Input: part model. Units: mm. Frame: model coordinates. A direction names the side the tool comes from. Give positions to 0.01 mm unless a question says otherwise; leave off trailing zeros. Loops run counter-clockwise (first coordinate to the right, second up) from the corner with the lowest first, then second, coordinate; pieces in that order, holes last. Notation, with made-up numbers: (56, 21) -> (75, 21) arc R20 cw to (75, 36) -> close; hole circle Ø5 at (85, 49.25). An arc over 180 degrees is marked (long way). Answer as a JSON object with one key per item and string values.
```python
from build123d import *

# Parameters (mm, degrees)
SKETCH1_R           = 60
BOSS_EXTRUDE1_DEPTH = 3
SKETCH2_R           = 7.4
CUT_EXTRUDE3_DEPTH  = 85.905830189
CUT_EXTRUDE1_START  = -3
SKETCH3_W           = 3
SKETCH3_H           = 65
CUT_EXTRUDE1_DEPTH  = 3
SKETCH4_W           = 5
SKETCH4_H           = 5
SKETCH4_W_2         = 5.5
SKETCH4_H_2         = 8.5
CUT_EXTRUDE2_DEPTH  = 3
SKETCH6_R           = 2
CUT_EXTRUDE4_DEPTH  = 77.896033708


with BuildPart() as part:
    # Sketch1 → Boss-Extrude1 (new body)
    with BuildSketch(Plane(origin=(0, 0, 0), x_dir=(1, 0, 0), z_dir=(0, 1, 0))):
        with Locations(Location((0, 0, 0), (0, 0, 270))):
            Circle(SKETCH1_R)
    extrude(amount=BOSS_EXTRUDE1_DEPTH)

    # Sketch2 → Cut-Extrude3 (cut, through all)
    with BuildSketch(Plane(origin=(0, 3, 0), x_dir=(1, 0, 0), z_dir=(0, 1, 0))):
        with Locations(Location((0, 0, 0), (0, 0, 270))):
            Circle(SKETCH2_R)
    extrude(amount=-CUT_EXTRUDE3_DEPTH, mode=Mode.SUBTRACT)

    # Sketch3 → Cut-Extrude1 (cut)
    with BuildSketch(Plane(origin=(0, 3, 0), x_dir=(1, 0, 0), z_dir=(0, 1, 0)).offset(CUT_EXTRUDE1_START)):
        with Locations((-46.5, 0)):
            Rectangle(SKETCH3_W, SKETCH3_H)
        with BuildLine():
            Line((-48, 32.5), (-48, 36))
            ThreePointArc((-48, 36), (-60, 0), (-48, -36))
            Line((-48, -36), (-48, -32.5))
            Line((-48, -32.5), (-48, 32.5))
        make_face()
    cut_extrude1 = extrude(amount=CUT_EXTRUDE1_DEPTH, mode=Mode.SUBTRACT)

    # Sketch4 → Cut-Extrude2 (cut)
    with BuildSketch(Plane(origin=(0, 3, 0), x_dir=(1, 0, 0), z_dir=(0, 1, 0))):
        Polygon((-40, 21.75), (-40, 20), (-40, 15), (-40, 13.25), (-34.5, 13.25), (-34.5, 21.75), align=None)
        with Locations((-42.5, 17.5)):
            Rectangle(SKETCH4_W, SKETCH4_H)
        with Locations((-37.25, -17.5)):
            Rectangle(SKETCH4_W_2, SKETCH4_H_2)
        with Locations((-42.5, -17.5)):
            Rectangle(SKETCH4_W, SKETCH4_H)
    cut_extrude2 = extrude(amount=-CUT_EXTRUDE2_DEPTH, mode=Mode.SUBTRACT)

    # Mirror1: Cut-Extrude1, Cut-Extrude2 across plane
    add(cut_extrude1.mirror(Plane(origin=(0, 0, 0), x_dir=(0, 0, 1), z_dir=(1, 0, 0))), mode=Mode.SUBTRACT)
    add(cut_extrude2.mirror(Plane(origin=(0, 0, 0), x_dir=(0, 0, 1), z_dir=(1, 0, 0))), mode=Mode.SUBTRACT)

    # Sketch6 → Cut-Extrude4 (cut, through all)
    with BuildSketch(Plane(origin=(0, 3, 0), x_dir=(1, 0, 0), z_dir=(0, 1, 0))):
        with Locations(Location((25.980762114, -15, 0), (0, 0, 270))):
            Circle(SKETCH6_R)
        with Locations(Location((0, 30, 0), (0, 0, 270))):
            Circle(SKETCH6_R)
        with Locations(Location((-25.980762114, -15, 0), (0, 0, 270))):
            Circle(SKETCH6_R)
    extrude(amount=-CUT_EXTRUDE4_DEPTH, mode=Mode.SUBTRACT)


solid = part.part
```
Q1. Access query for faces 1 (the flat face through (-45, 1, 0)), 2 (the flat face through (11, 0, -1)), 3 (the flat face through (-48, 1, -34)), 4 (the flat face through (43, 2, -15)), 5 (the flat face through (37, 2, 21.75)). Directions: +Z, -Z, +X, -X, +Y, -Y. A direction counts if a zero-diameter tool reaches every point of the face in a straight line with its end or side. Return the directions, or none.
Evaluation:
{"face 1": "-X, +Y, -Y", "face 2": "+Z, -Z, +X, -X, -Y", "face 3": "+Z, -Z, -X, +Y, -Y", "face 4": "+X, +Y, -Y", "face 5": "+Y, -Y"}
Q2. Ray query, line 1 along Z through (x, y) = (37, 0.3); line 2 along Z through (x, y) = (38, 0.85); line 3 along X through (y, z) = (2.3, -30). Return the intervals inside material, ascending.
Evaluation:
{"line 1": "z = -47.23 to -21.75, -13.25 to 13.25, 21.75 to 47.23", "line 2": "z = -46.43 to -21.75, -13.25 to 13.25, 21.75 to 46.43", "line 3": "x = -45 to -2, 2 to 45"}
Q3. Pin query (flat end, axial travel): pin 1 (0.9 mm diameter, centred on x = 46, y = 1, fed in from -Z); pin 2 (1.5 mm diameter, centred on y = 2, z = -0.5, fed in from +X); pin 3 (1.5 mm diameter, centred on x = 41.5, y = 2, fed in from +Z). Return the tip coordinate at first contact, or that it passes through.
Evaluation:
{"pin 1": "stops at z = -39.05", "pin 2": "stops at x = 45", "pin 3": "stops at z = 44.04"}
Q4. Section A-A, the plane z = 0. Return the cut outline in (x, y), then the cut area to 3 significant figures.
Evaluation:
{"outline": "(-45, 0) -> (-7.4, 0) -> (-7.4, 3) -> (-45, 3) -> close; (7.4, 0) -> (45, 0) -> (45, 3) -> (7.4, 3) -> close", "area": "226 mm2"}
Q5. Section D-D, the plane z = 18.5. Return the cut outline in (x, y).
Evaluation:
{"outline": "(-34.5, 0) -> (34.5, 0) -> (34.5, 3) -> (-34.5, 3) -> close"}
Q6. Section B-B, the plane x = 36.5. Return the cut outline in (y, z).
Evaluation:
{"outline": "(0, -47.62) -> (3, -47.62) -> (3, -21.75) -> (0, -21.75) -> close; (0, -13.25) -> (3, -13.25) -> (3, 13.25) -> (0, 13.25) -> close; (0, 21.75) -> (3, 21.75) -> (3, 47.62) -> (0, 47.62) -> close"}
Q7. Section C-C, the plane z = -30. Return the cut outline in (x, y), then the cut area to 3 significant figures.
Evaluation:
{"outline": "(-45, 0) -> (-2, 0) -> (-2, 3) -> (-45, 3) -> close; (2, 0) -> (45, 0) -> (45, 3) -> (2, 3) -> close", "area": "258 mm2"}
Q8. Draft query along X for faces 6 (the flat face through (-48, 1, 34)), 7 (the flat face through (37, 2, -13.25)), 8 (the flat face through (45, 1, 0)), 9 (the flat face through (-37, 2, 21.75)). Return one class per face: +X half, -X half, draft (parallel to the pull), parting line (faces both ways), or undercut.
Evaluation:
{"face 6": "-X half", "face 7": "undercut", "face 8": "+X half", "face 9": "undercut"}
